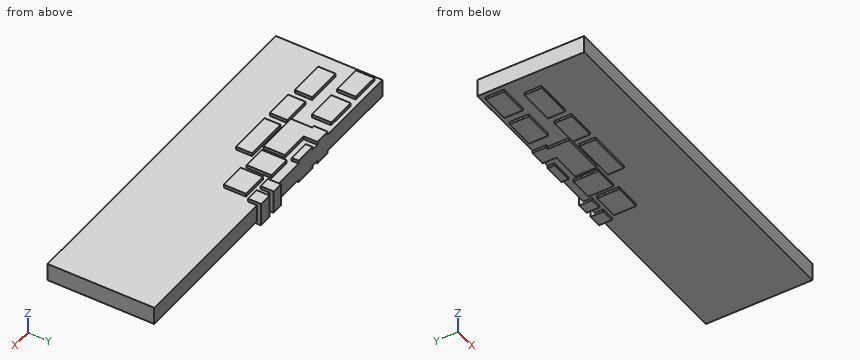
```python
from build123d import *

# Parameters (mm, degrees)
F0_W          = 100
F0_H          = 30
F1_DEPTH      = 5
F2_W          = 8.196883
F2_H          = 5.239555
F2_W_2        = 10.289293
F2_H_2        = 4.854159
F2_W_3        = 8.500245
F2_H_3        = 5.465182
F2_W_4        = 8.03056
F2_H_4        = 4.854797
F2_W_5        = 12.510864
F2_H_5        = 4.473866
F2_W_6        = 6.646618
F2_H_6        = 7.028431
F2_W_7        = 6.090546
F2_H_7        = 1.946411
F2_W_8        = 7.445213
F2_H_8        = 6.23659
F2_W_9        = 3.194372
F2_H_9        = 3.654776
F2_W_10       = 3.732365
F3_DEPTH      = 0.9
F3_DEPTH_BACK = 5.7


with BuildPart() as f1:
    # F0 (on Top) → F1 (new body)
    with BuildSketch(Plane.XY):
        with Locations((-11.689384, -8.387734)):
            Rectangle(F0_W, F0_H)
    extrude(amount=F1_DEPTH)

    # F2 (on face) → F3 (join, two sides)
    with BuildSketch(Plane.XY.offset(5)) as f3_sk:
        with Locations((-56.269321, 2.619778)):
            Rectangle(F2_W, F2_H)
        with Locations((-51.577137, -5.787824)):
            Rectangle(F2_W_2, F2_H_2)
        with Locations((-45.274136, 2.732591)):
            Rectangle(F2_W_3, F2_H_3)
        Polygon((-37.700053, 2.719443), (-36.987849, 2.719443), (-33.169098, 2.719443), (-33.169098, 6.612266), (-37.700053, 6.612266), align=None)
        Polygon((-33.169098, 2.719443), (-36.987849, 2.719443), (-36.987849, -3.260119), (-24.9527, -3.260119), (-24.9527, 2.719443), align=None)
        with Locations((-40.126903, -6.190432)):
            Rectangle(F2_W_4, F2_H_4)
        with Locations((-27.565886, -6.402896)):
            Rectangle(F2_W_5, F2_H_5)
        with Locations((-20.288212, 0.609834)):
            Rectangle(F2_W_6, F2_H_6)
        with Locations((-27.997973, 5.63906)):
            Rectangle(F2_W_7, F2_H_7)
        with Locations((-11.670222, -0.398852)):
            Rectangle(F2_W_8, F2_H_8)
        with Locations((-13.795643, 5.951438)):
            Rectangle(F2_W_9, F2_H_9)
        with Locations((-8.564607, 5.951438)):
            Rectangle(F2_W_10, F2_H_9)
    extrude(amount=F3_DEPTH)
    extrude(f3_sk.sketch, amount=-F3_DEPTH_BACK)


solid = f1.part
```
Can you work these out from the model? Positions are in its coordinate system, mm. Coordinates: 2 decimals unless noted, no trailing zeros. Loops run counter-clockwise (first coordinate to the right, second up) from the corner with the lowest first, then second, coordinate; pieces in that order, holes last. Notation, with made-up numbers: M -7,-19 L 18,-19 A28 cw 18,13 Z; hole C 31,-35 d3. An arc over 180 degrees is marked long. Put each result on its own line as item: value. Start each with the question number.
(1) Imagine slicing it at B-B on x = 31.5. List the corners of the cut face in (y, z) for me.
(2) Will these pins go through, and if not, where does the flat tip stop? pin 1 Ø5 at (x, y) = (-40, -16.5) entering from +Z; pin 2 Ø5 at (x, y) = (-1, 1) entering from -Z; pin 3 Ø0.7 at (y, z) = (-4.5, 5.5) entering from +X.
(3) Imagine slicing it at A-A on z = 4. List the corners of the cut face in (x, y) for me, and give its area (3 significant figures).
(4) Imagine slicing it at C-C on y = -16. List the corners of the cut face in (x, z) for me.
(5) I need wall thicknesses on probe 1 along Y at (x, z) = (-47.5, 5.75); probe 2 along Y at (x, z) = (-18, 1); probe 3 along Z at (x, y) = (-0.5, 0). Which ranges of each line are inside material? Lowest first, please.
Worked answers:
1. outline: M -23.39,0 L 6.61,0 L 6.61,5 L -23.39,5 Z
2. pin 1: stops at z = 5
2. pin 2: stops at z = 0
2. pin 3: stops at x = -21.31
3. outline: M -61.69,-23.39 L 38.31,-23.39 L 38.31,6.61 L -6.7,6.61 L -6.7,7.78 L -10.43,7.78 L -10.43,6.61 L -12.2,6.61 L -12.2,7.78 L -15.39,7.78 L -15.39,6.61 L -61.69,6.61 Z
3. area: 3,010 mm2
4. outline: M -61.69,0 L 38.31,0 L 38.31,5 L -61.69,5 Z
5. probe 1: y = -8.21 to -3.36, 0 to 5.47
5. probe 2: y = -23.39 to 6.61
5. probe 3: z = 0 to 5
